For this review, take the finished solid that the model builds, in its own axes (mm). A direction names the side the tool comes from. Give positions to 0.01 mm unless a question says otherwise; leave off trailing zeros. Order: outer loops, then holes, each group sorted by start corner. A loop starts at its lowest first (then second) coordinate and runs counter-clockwise, first axis right, second up.
from build123d import *

# Parameters (mm, degrees)
SKETCH001_W     = 156
SKETCH001_H     = 50.32
PAD_DEPTH       = 1.5
SKETCH004_W     = 17.5
SKETCH004_H     = 17.5
PAD001_DEPTH    = 3.5
SKETCH005_R     = 3.7
SKETCH005_W     = 14.5
SKETCH005_H     = 14.5
POCKET_DEPTH    = 5
SKETCH007_W     = 14.19
SKETCH007_H     = 16.92
SKETCH007_W_2   = 17.17
SKETCH007_H_2   = 38.96
POCKET001_DEPTH = 5


with BuildPart() as part:
    # Sketch001 → Pad (new body)
    with BuildSketch(Plane.XY):
        with Locations((121, -79.51)):
            Rectangle(SKETCH001_W, SKETCH001_H)
    extrude(amount=PAD_DEPTH)

    # Sketch004 (on DatumPlane) → Pad001 (join)
    with BuildSketch(Plane(origin=(0, 0, 0), x_dir=(1, 0, 0), z_dir=(0, 0, -1))):
        with Locations((51.75, 64)):
            Rectangle(SKETCH004_W, SKETCH004_H)
        with Locations((74.75, 64)):
            Rectangle(SKETCH004_W, SKETCH004_H)
        with Locations((97.75, 64)):
            Rectangle(SKETCH004_W, SKETCH004_H)
        with Locations((120.75, 64)):
            Rectangle(SKETCH004_W, SKETCH004_H)
        with Locations((143.75, 64)):
            Rectangle(SKETCH004_W, SKETCH004_H)
        with Locations((166.75, 64)):
            Rectangle(SKETCH004_W, SKETCH004_H)
        with Locations((189.75, 64)):
            Rectangle(SKETCH004_W, SKETCH004_H)
        with Locations((63.25, 96.5)):
            Rectangle(SKETCH004_W, SKETCH004_H)
        with Locations((86.25, 96.5)):
            Rectangle(SKETCH004_W, SKETCH004_H)
        with Locations((109.25, 96.5)):
            Rectangle(SKETCH004_W, SKETCH004_H)
        with Locations((155.25, 96.5)):
            Rectangle(SKETCH004_W, SKETCH004_H)
        with Locations((178.25, 96.5)):
            Rectangle(SKETCH004_W, SKETCH004_H)
    extrude(amount=PAD001_DEPTH)

    # Sketch005 (on DatumPlane) → Pocket (cut)
    with BuildSketch(Plane.XY.offset(1.5)):
        with Locations((114, -109)):
            Circle(SKETCH005_R)
        with Locations((51.75, -64)):
            Rectangle(SKETCH005_W, SKETCH005_H)
        with Locations((74.75, -64)):
            Rectangle(SKETCH005_W, SKETCH005_H)
        with Locations((97.75, -64)):
            Rectangle(SKETCH005_W, SKETCH005_H)
        with Locations((120.75, -64)):
            Rectangle(SKETCH005_W, SKETCH005_H)
        with Locations((143.75, -64)):
            Rectangle(SKETCH005_W, SKETCH005_H)
        with Locations((166.75, -64)):
            Rectangle(SKETCH005_W, SKETCH005_H)
        with Locations((189.75, -64)):
            Rectangle(SKETCH005_W, SKETCH005_H)
        with Locations((63.25, -96.5)):
            Rectangle(SKETCH005_W, SKETCH005_H)
        with Locations((86.25, -96.5)):
            Rectangle(SKETCH005_W, SKETCH005_H)
        with Locations((109.25, -96.5)):
            Rectangle(SKETCH005_W, SKETCH005_H)
        with Locations((155.25, -96.5)):
            Rectangle(SKETCH005_W, SKETCH005_H)
        with Locations((178.25, -96.5)):
            Rectangle(SKETCH005_W, SKETCH005_H)
    extrude(amount=-POCKET_DEPTH, mode=Mode.SUBTRACT)

    # Sketch007 → Pocket001 (cut)
    with BuildSketch(Plane.XY.offset(1.5)):
        with Locations((45.095, -100.46)):
            Rectangle(SKETCH007_W, SKETCH007_H)
        with Locations((199.265, -93.9)):
            Rectangle(SKETCH007_W_2, SKETCH007_H_2)
    extrude(amount=-POCKET001_DEPTH, mode=Mode.SUBTRACT)


solid = part.part
1) Draft analysis for pull direction Y (two halves, no side actions). For faces 1 (the face through (198.5, -64, -2)), 2 (the face through (171, -97, -1)), 3 (the face through (86, -87.75, -2)), 4 (the face through (167, -55.25, -2)), state which applies: +Y half, -Y half, draft (parallel to the pull), parting line (faces both ways), or undercut.
Answer sheet:
face 1: draft
face 2: undercut
face 3: undercut
face 4: +Y half
2) Clearance check with flat-ended pins moving along their axes: pin 1 (1.6 mm diameter, centred on y = -90, z = 1, fed in from +X); pin 2 (1.5 mm diameter, centred on x = 128.5, z = -2, fed in from +Y); pin 3 (1.5 mm diameter, centred on x = 100, z = -1, fed in from -Y); pin 4 (1.8 mm diameter, centred on y = -99.5, z = -1.5, fed in from -X). State where each tip first meets the part, or that it passes through.
Answer sheet:
pin 1: stops at x = 190.68
pin 2: stops at y = -55.25
pin 3: stops at y = -105.25
pin 4: stops at x = 54.5
3) To check wall thickness, follow line 1 (X direction, y = -89.5, z = 0.25); line 2 (Y direction, x = 114.5, z = -3); line 3 (Y direction, x = 171.5, z = 1.15). State the ranges of each line that lie inside material, in increasing order.
Answer sheet:
line 1: x = 43 to 56, 70.5 to 79, 93.5 to 102, 116.5 to 148, 162.5 to 171, 185.5 to 190.68
line 2: y = -105.25 to -103.75, -89.25 to -87.75, -72.75 to -71.25, -56.75 to -55.25
line 3: y = -104.67 to -103.75, -89.25 to -71.25, -56.75 to -54.35
4) We need section D-D on y = -78.5. Give the boundary of the cut face in (x, z), then the cut area to 3 significant figures.
Answer sheet:
outline: (43, 0) - (190.68, 0) - (190.68, 1.5) - (43, 1.5) - close
area: 222 mm2
5) Tool access review of faces 5 (the face through (164, -96, -2)), 6 (the face through (121, -56.75, -1)), 7 (the face through (75, -72.75, -2)), 8 (the face through (158, -64, -2)): name each direction out of +Z, -Z, +X, -X, +Y, -Y from which nothing blocks a thin tool from reaching the whole face with its end or side.
Answer sheet:
face 5: -Z, -Y
face 6: +Z, -Z
face 7: -Z, +X, -X
face 8: -Z, +Y
6) We need section B-B on z = -1.25. Count the separate pieces of the cut face and the enclosed holes in it, then the cut area to 3 significant figures.
Answer sheet:
separate pieces: 12
enclosed holes: 12
area: 1,150 mm2
7) We need section A-A on x = 145. Give the boundary of the cut face in (y, z), then the cut area to 3 significant figures.
Answer sheet:
outline: (-104.67, 0) - (-72.75, 0) - (-72.75, -3.5) - (-71.25, -3.5) - (-71.25, 1.5) - (-104.67, 1.5) - close; (-56.75, -3.5) - (-55.25, -3.5) - (-55.25, 0) - (-54.35, 0) - (-54.35, 1.5) - (-56.75, 1.5) - close
area: 64.2 mm2
